Autodesk Inventor part; units mm, degrees
ref_plane "YZ Plane" through (0, 0, 0) normal (1, 0, 0) x (0, 1, 0)
ref_plane "XZ Plane" through (0, 0, 0) normal (0, 1, 0) x (-1, 0, 0)
ref_plane "XY Plane" through (0, 0, 0) normal (0, 0, 1) x (1, 0, 0)
sketch "Sketch1" plane through (0, 0, 0) normal (0, 0, 1) x (1, 0, 0)
  line L0 (-12.7, -25.4) -> (12.7, -25.4)
  line L1 (12.7, -25.4) -> (12.7, 25.4)
  line L2 (12.7, 25.4) -> (-12.7, 25.4)
  line L3 (-12.7, 25.4) -> (-12.7, -25.4)
  line L4 (-12.7, -25.4) -> (12.7, 25.4) construction
  line L5 (12.7, -25.4) -> (-12.7, 25.4) construction
  line L6 (-11.1125, 23.8125) -> (11.1125, 23.8125)
  line L7 (11.1125, 23.8125) -> (11.1125, -23.8125)
  line L8 (11.1125, -23.8125) -> (-11.1125, -23.8125)
  line L9 (-11.1125, -23.8125) -> (-11.1125, 23.8125)
  point P0 (0, 0)
  dimension "width" = 25.4
  dimension "height" = 50.8
  dimension "thickness" = 1.5875
extrude "Extrusion1" add sketch "Sketch1" along normal mid plane 152.4
sketch "Sketch2" plane through (-12.7, 25.4, 76.2) normal (0, 1, 0) x (1, 0, 0)
  line L0 (0, 152.4) -> (0, 0) construction
  line L1 (25.4, 0) -> (0, 0) construction
  line L2 (25.4, 152.4) -> (25.4, 0) construction
  line L3 (0, 152.4) -> (25.4, 152.4) construction
  line L4 (12.7, 127) -> (12.7, 25.4) construction
  point P0 (12.7, 76.2)
  point P1 (12.7, 76.2)
  point P2 (12.7, 76.2)
  dimension "d5" = 101.6
hole "Hole1" at (0, 25.4, -50.8) at (0, 25.4, 50.8) at (0, 25.4, 0) direction (0, -1, 0) diameter 5.1054 end through all
sketch "Sketch4" plane through (12.7, -25.4, 76.2) normal (1, 0, 0) x (0, 0, -1)
  circle A0 centre (76.2, 25.4) radius 53.75 construction
  line L0 (25.9391, 6.35) -> (126.4609, 6.35) construction
  line L1 (126.4609, 6.35) -> (126.4609, 44.45) construction
  line L2 (126.4609, 44.45) -> (25.9391, 44.45) construction
  line L3 (25.9391, 44.45) -> (25.9391, 6.35) construction
  line L4 (25.9391, 6.35) -> (126.4609, 44.45) construction
  line L5 (126.4609, 6.35) -> (25.9391, 44.45) construction
  line L6 (0, 0) -> (0, 50.8) construction
  dimension "d25" = 107.5
  dimension "d28" = 38.1
hole "Hole3" at (12.7, 19.05, 50.2609) at (12.7, 19.05, -50.2609) at (12.7, -19.05, -50.2609) at (12.7, -19.05, 50.2609) direction (-1, 0, 0) diameter 5.1054 end through all
sketch "Sketch5" plane through (-12.7, 25.4, 76.2) normal (0, 1, 0) x (1, 0, 0)
  line L0 (25.4, 0) -> (0, 0)
  line L1 (12.7, 136.525) -> (12.7, 15.875) construction
  line L2 (0, 152.4) -> (0, 0) construction
  point P0 (12.7, 76.2)
  point P1 (12.7, 0)
  point P2 (12.7, 76.2)
  point P3 (0, 76.2)
  dimension "d36" = 120.65
hole "Hole4" at (0, 25.4, -60.325) at (0, 25.4, 60.325) direction (0, -1, 0) diameter 5.1054 end through all
sketch "Sketch3" plane through (12.7, -25.4, 76.2) normal (1, 0, 0) x (0, 0, -1)
  line L0 (25.9391, 44.45) -> (126.4609, 44.45) construction
  line L1 (126.4609, 44.45) -> (126.4609, 6.35) construction
  line L2 (126.4609, 6.35) -> (25.9391, 6.35) construction
  line L3 (25.9391, 6.35) -> (25.9391, 44.45) construction
  line L4 (25.9391, 44.45) -> (126.4609, 6.35) construction
  line L5 (126.4609, 44.45) -> (25.9391, 6.35) construction
  circle A0 centre (76.2, 25.4) radius 60 construction
  circle A1 centre (76.2, 25.4) radius 47.5 construction
  circle A2 centre (76.2, 25.4) radius 53.75 construction
  dimension "d16" = 107.5
  dimension "d14" = 120
  dimension "d15" = 95
  dimension "d17" = 38.1
properties part number "GP9-004" material "Aluminum 6061"
Work out the finished part from the listing and answer in its coordinate system (mm). A direction names the side the tool comes from. Round coordinates to 2 decimals unless told otherwise and drop trailing zeros. Write each loop counter-clockwise with the first axis right and the second up, starting at its lowest first coordinate (ties: lowest second). Pieces come first, ordered by that corner, then holes. Notation, with made-up numbers: (53, -37) -> (102, -37) arc R9 cw to (102, -30) -> close; hole circle Ø6 at (4, -20). An arc over 180 degrees is marked (long way). Write each question's results on one line, items separated by ' | '.
Item 1: A cutting plane is placed at B-B, the plane z = 0. Determine the outline of the cut face in (x, y), plus the area to 3 significant figures.
Result set:
outline: (-12.7, -25.4) -> (-2.55, -25.4) -> (-2.55, -23.81) -> (-11.11, -23.81) -> (-11.11, 23.81) -> (-2.55, 23.81) -> (-2.55, 25.4) -> (-12.7, 25.4) -> close; (2.55, -25.4) -> (12.7, -25.4) -> (12.7, 25.4) -> (2.55, 25.4) -> (2.55, 23.81) -> (11.11, 23.81) -> (11.11, -23.81) -> (2.55, -23.81) -> close | area: 216 mm^2
Item 2: A cutting plane is placed at D-D, the plane z = -39.5. Determine the outline of the cut face in (x, y), plus the area to 3 significant figures.
Result set:
outline: (-12.7, -25.4) -> (12.7, -25.4) -> (12.7, 25.4) -> (-12.7, 25.4) -> close; hole (-11.11, -23.81) -> (11.11, -23.81) -> (11.11, 23.81) -> (-11.11, 23.81) -> close | area: 232 mm^2
Item 3: A cutting plane is placed at A-A, the plane y = 19.05. Determine the outline of the cut face in (x, z).
Result set:
outline: (-12.7, -76.2) -> (-11.11, -76.2) -> (-11.11, -52.81) -> (-12.7, -52.81) -> close; (-12.7, -47.71) -> (-11.11, -47.71) -> (-11.11, 47.71) -> (-12.7, 47.71) -> close; (-12.7, 52.81) -> (-11.11, 52.81) -> (-11.11, 76.2) -> (-12.7, 76.2) -> close; (11.11, -76.2) -> (12.7, -76.2) -> (12.7, -52.81) -> (11.11, -52.81) -> close; (11.11, -47.71) -> (12.7, -47.71) -> (12.7, 47.71) -> (11.11, 47.71) -> close; (11.11, 52.81) -> (12.7, 52.81) -> (12.7, 76.2) -> (11.11, 76.2) -> close
Item 4: Which of the six approach directions +Z, -Z, +X, -X, +Y, -Y give full straight-line access (tool end or side, diameter ignored) to faces 4 (the face through (-3, 23.812, -1)), 5 (the face through (-0.767, 24.595, 2.435))?
Result set:
face 4: +Z, -Z | face 5: +Y, -Y
Item 5: Find the intervals of material crossed by line 1 along Z through (x, y) = (-12.05, 19.05); line 2 along Z through (x, y) = (0, 25); line 3 along X through (y, z) = (-19.5, 34), in increasing order. Write a range as [from, to].
Result set:
line 1: [-76.2, -52.81], [-47.71, 47.71], [52.81, 76.2] | line 2: [-76.2, -62.88], [-57.77, -53.35], [-48.25, -2.55], [2.55, 48.25], [53.35, 57.77], [62.88, 76.2] | line 3: [-12.7, -11.11], [11.11, 12.7]
Item 6: The mould has two halves that part along X. Classify faces 1 (the face through (12.7, 0, -1)), 2 (the face through (-11.917, -16.558, 50.814)), 3 (the face through (-0.112, -24.617, -62.875)): +X half, -X half, draft (parallel to the pull), parting line (faces both ways), or undercut.
Result set:
face 1: +X half | face 2: draft | face 3: undercut
Item 7: A cutting plane is placed at C-C, the plane x = 5.25. Determine the outline of the cut face in (y, z).
Result set:
outline: (-25.4, -76.2) -> (-23.81, -76.2) -> (-23.81, 76.2) -> (-25.4, 76.2) -> close; (23.81, -76.2) -> (25.4, -76.2) -> (25.4, 76.2) -> (23.81, 76.2) -> close
